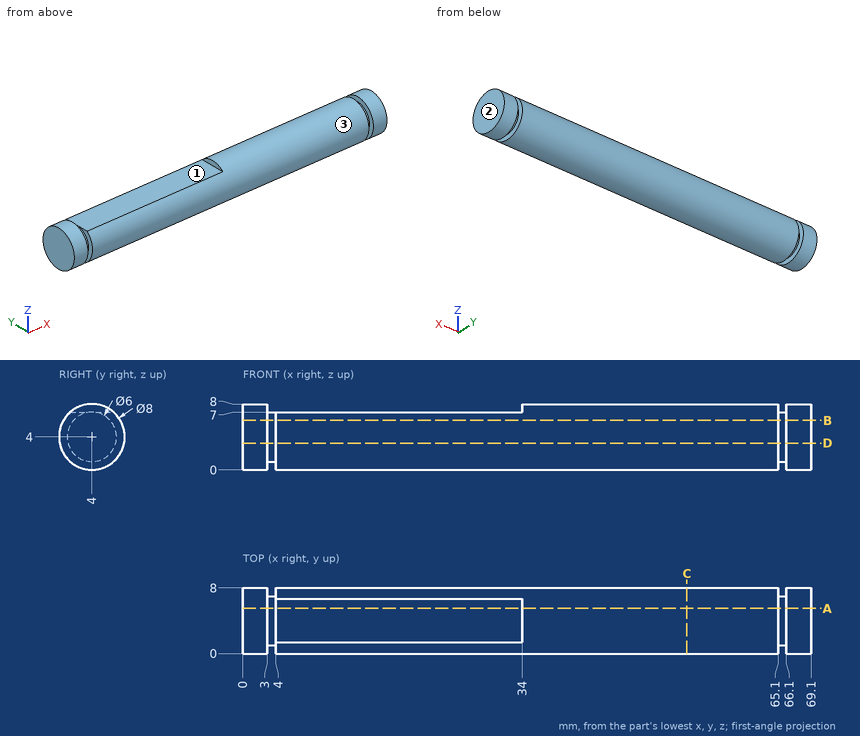
Design review of the part shown in the three views and the two pictorial views. Dimensions are in mm from the part's minimum x, y and z. Round coordinates to 2 decimals unless told otherwise and drop trailing zeros. Loops run counter-clockwise (first coordinate to the right, second up) from the corner with the lowest first, then second, coordinate; pieces in that order, holes last. Notation, with made-up numbers: (9, 50) - (27, 50) arc R29 cw to (27, 81) - close; hole circle Ø6 at (-4, 62.5). An arc over 180 degrees is marked (long way). Write each question's results on one line, items separated by ' | '. Start each with the question number.
Q1. Take a section at C-C on x = 54. Give the boundary of the cut face in (y, z), plus the area to 3 significant figures.
Q2. Insertion check: P1, Ø1, axis at x = 35, y = 3, coming from the -Z side; P2, Ø4, axis at x = 15, y = 3.5, coming from the +Z side. Each pin has a flat end and moves straight along its axis. Give the tip position at first contact, or say it passes through.
Q3. Take a section at A-A on y = 5.5. Give the boundary of the cut face in (x, z), plus the area to 3 significant figures.
Q4. Wall thickness on line 1 along X through (y, z) = (1.5, 6.5); line 2 along X through (y, z) = (4.25, 7.5); line 3 along Y through (x, z) = (14, 4.25): over which ranges is each line inside the solid? List them lowest first. Write a range as [from, to].
Q5. Take a section at B-B on z = 6. Give the boundary of the cut face in (x, y), plus the area to 3 significant figures.
Q6. Take a section at D-D on z = 3.25. Give the boundary of the cut face in (x, y).
Q7. Draft analysis for pull direction X (two halves, no side actions). For the marked faces 1, 2 and 3, state which applies: pulls with the +X half, pulls with the -X half, needs draft (parallel to the pull), parting line crosses it, or undercut.
Data:
1) outline: circle Ø8 at (4, 4) | area: 50.3 mm²
2) P1: stops at z = 0.03 | P2: stops at z = 7
3) outline: (0, 0.29) - (3, 0.29) - (3, 1.4) - (4, 1.4) - (4, 0.29) - (65.1, 0.29) - (65.1, 1.4) - (66.1, 1.4) - (66.1, 0.29) - (69.1, 0.29) - (69.1, 7.71) - (66.1, 7.71) - (66.1, 6.6) - (65.1, 6.6) - (65.1, 7.71) - (34, 7.71) - (34, 7) - (4, 7) - (4, 6.6) - (3, 6.6) - (3, 7.71) - (0, 7.71) - close | area: 487 mm²
4) line 1: x = [0, 3], [4, 65.1], [66.1, 69.1] | line 2: x = [0, 3], [34, 65.1], [66.1, 69.1] | line 3: y = [0.01, 7.99]
5) outline: (0, 0.54) - (3, 0.54) - (3, 1.76) - (4, 1.76) - (4, 0.54) - (65.1, 0.54) - (65.1, 1.76) - (66.1, 1.76) - (66.1, 0.54) - (69.1, 0.54) - (69.1, 7.46) - (66.1, 7.46) - (66.1, 6.24) - (65.1, 6.24) - (65.1, 7.46) - (4, 7.46) - (4, 6.24) - (3, 6.24) - (3, 7.46) - (0, 7.46) - close | area: 474 mm²
6) outline: (0, 0.07) - (3, 0.07) - (3, 1.1) - (4, 1.1) - (4, 0.07) - (65.1, 0.07) - (65.1, 1.1) - (66.1, 1.1) - (66.1, 0.07) - (69.1, 0.07) - (69.1, 7.93) - (66.1, 7.93) - (66.1, 6.9) - (65.1, 6.9) - (65.1, 7.93) - (4, 7.93) - (4, 6.9) - (3, 6.9) - (3, 7.93) - (0, 7.93) - close
7) face 1: undercut | face 2: pulls with the +X half | face 3: needs draft
